For this review, take the finished solid that the model builds, in its own axes (mm). A direction names the side the tool comes from. Coordinates: 2 decimals unless noted, no trailing zeros. Loops run counter-clockwise (first coordinate to the right, second up) from the corner with the lowest first, then second, coordinate; pieces in that order, holes last. Notation, with made-up numbers: M 0,86 L 11,86 A14 cw 11,109 Z; hole C -17.5,44.5 d11. An arc over 180 degrees is marked long. Write item = value, one per line.
from build123d import *

# Parameters (mm, degrees)
F0_W      = 82
F0_H      = 36
F1_DEPTH  = 7.7
F2_W      = 82
F2_H      = 54
F3_DEPTH  = 7.2
F4_R      = 7.4840620434
F5_R      = 5
F6_W      = 6.2068961561
F6_H      = 3.4913793206
F7_DEPTH  = 0.8
F10_DEPTH = 4
F11_DEPTH = 4
F12_W     = 81.9998856485
F12_H     = 29.2846155894
F13_DEPTH = 1.1


with BuildPart() as f1:
    # F0 (on Front) → F1 (new body)
    with BuildSketch(Plane.XZ):
        Rectangle(F0_W, F0_H)
    extrude(amount=F1_DEPTH)

    # F2 (on face) → F3 (join)
    with BuildSketch(Plane.XY.offset(18)):
        with Locations((0, 19.672181885)):
            Rectangle(F2_W, F2_H)
    extrude(amount=-F3_DEPTH)

    # F4
    f4_edges = [f1.edges().sort_by_distance(p)[0] for p in [
        (41, 19.486091, 18),
        (-41, 19.486091, 18),
    ]]
    fillet(f4_edges, radius=F4_R)

    # F5
    f5_edges = [f1.edges().sort_by_distance(p)[0] for p in [
        (-41, -3.85, -18),
        (41, -3.85, -18),
    ]]
    fillet(f5_edges, radius=F5_R)

    # F6 (on face) → F7 (join)
    with BuildSketch(Plane.XZ.offset(7.7)):
        with Locations((-25.83758533, 6.2539605424)):
            Rectangle(F6_W, F6_H)
        with Locations((25.83758533, 6.2539605424)):
            Rectangle(F6_W, F6_H)
    extrude(amount=F7_DEPTH)

    # F8 (on face) → F10 (join)
    with BuildSketch(Plane.YZ.offset(41)):
        with BuildLine():
            Line((46.3586388528, 11.4392106599), (0, 11.4392106599))
            Line((0, 11.4392106599), (0, 10.5159379566))
            Line((0, 10.5159379566), (0, -13))
            Line((0, -13), (0, -18.1146790814))
            Line((0, -18.1146790814), (14.7262415299, -18.1146790814))
            ThreePointArc((14.7262415299, -18.1146790814), (30.5080702528, -5.8071597095), (46.2898989758, -18.1146790814))
            Line((46.2898989758, -18.1146790814), (46.3586388528, -18.1146790814))
            Line((46.3586388528, -18.1146790814), (46.3586388528, 11.4392106599))
        make_face()
    extrude(amount=-F10_DEPTH)

    # F9 (on face) → F11 (join)
    with BuildSketch(Plane(origin=(-41, 0, 0), x_dir=(0, -1, 0), z_dir=(-1, 0, 0))):
        with BuildLine():
            Line((0, 10.5159379566), (0, 11.1698398332))
            Line((0, 11.1698398332), (-47.3828552663, 11.1698398332))
            Line((-47.3828552663, 11.1698398332), (-47.3828552663, -16.3062599394))
            ThreePointArc((-47.3828552663, -16.3062599394), (-29.7853048283, -4.7156749244), (-13.1738176833, -17.6800081985))
            Line((-13.1738176833, -17.6800081985), (0, -17.6800081985))
            Line((0, -17.6800081985), (0, -13))
            Line((0, -13), (0, 10.5159379566))
        make_face()
    extrude(amount=-F11_DEPTH)

    # F12 (on face) + F3_face2 (on face) → F13 (join)
    with BuildSketch(Plane(origin=(0, 46.3586388528, 0), x_dir=(-1, 0, 0), z_dir=(0, 1, 0))):
        with Locations((-5.71758e-05, -3.4723712868)):
            Rectangle(F12_W, F12_H)
    with BuildSketch(Plane(origin=(0.1017201648, 46.672181885, 14.3268391262), x_dir=(-1, 0, 0), z_dir=(0, 1, 0))):
        with BuildLine():
            Line((33.6176581214, 3.6731608738), (-33.4142177919, 3.6731608738))
            ThreePointArc((-33.4142177919, 3.6731608738), (-38.6048462082, 1.5806256376), (-40.8928870201, -3.5268391262))
            Line((-40.8928870201, -3.5268391262), (37.1017201648, -3.5268391262))
            Line((37.1017201648, -3.5268391262), (37.1017201648, -3.156999293))
            Line((37.1017201648, -3.156999293), (41.0730988867, -3.156999293))
            ThreePointArc((41.0730988867, -3.156999293), (38.67321657, 1.7074784333), (33.6176581214, 3.6731608738))
        make_face()
    extrude(amount=F13_DEPTH)


solid = f1.part
Q1. For pin 1 Ø8.5 at (x, z) = (-12.5, -8) entering from -Y; pin 2 Ø4 at (x, y) = (10, 11) entering from -Z; pin 3 Ø4 at (x, z) = (-13, -11) entering from +Y, all flat-tipped, find the tip position at first contact; note any pin that passes through.
Solved:
pin_1 = -7.7
pin_2 = 10.8
pin_3 = 47.46
Q2. For line 1 along Y through (x, z) = (25.5, 3.5); line 2 along X through (y, z) = (2.5, -14); line 3 along Z through (x, y) = (31, 4), list the stretches that pass through material, from the lowest coordinate up.
Solved:
line_1 = -7.7 to 0, 46.36 to 47.46
line_2 = -41 to -37, 37 to 41
line_3 = 10.8 to 18
Q3. Draft analysis for pull direction Y (two halves, no side actions). For faces 1 (the face through (0, 20, 18)), 2 (the face through (-1, 24, 10.8)), 3 (the face through (-40, 0, -17)), state which applies: +Y half, -Y half, draft (parallel to the pull), parting line (faces both ways), or undercut.
Solved:
face_1 = draft
face_2 = undercut
face_3 = -Y half
Q4. Machinability: for faces 4 (the face through (-39, 25.2, -5.5)), 5 (the face through (-40, -4, -16)), 6 (the face through (39, -4, -17)), 7 (the face through (-1, 0, -3)), which of the approach directions +Z, -Z, +X, -X, +Y, -Y give a long, thin tool a straight path to every point of the face, cutting with its end or side? Answer none if there is none.
Solved:
face_4 = -Z, -X
face_5 = -Z, -X, -Y
face_6 = -Z, +X, -Y
face_7 = -Z
Q5. Add section C-C (x = -2). Write out the cut boundary in (y, z), and give its area (3 significant figures).
Solved:
outline = M -7.7,-18 L 0,-18 L 0,10.8 L 46.36,10.8 L 46.36,-18.11 L 47.46,-18.11 L 47.46,10.8 L 47.77,10.8 L 47.77,18 L -7.7,18 Z
area = 653 mm²
Q6. Add section D-D (z = 14). Write out the cut boundary in (x, y).
Solved:
outline = M -40.14,-7.7 L 40.14,-7.7 L 40.14,47.77 L -40.14,47.77 Z
